Can you work these out from the drawing? Everything is in mm from the part's minimum corner. A direction names the side the tool comes from. Give positions to 0.01 mm unless a question says otherwise; leave off trailing zeros. Order: outer loops, then holes, each group sorted by start corner. A loop starts at its lowest first (then second) coordinate and runs counter-clockwise, first axis right, second up. Notation, with made-up numbers: (12, 20.25) - (16, 20.25) arc R26 cw to (16, 40.25) - close; hole circle Ø9 at (21, -2). An arc over 180 degrees is marked (long way). One line per question, with ' | ' between items.
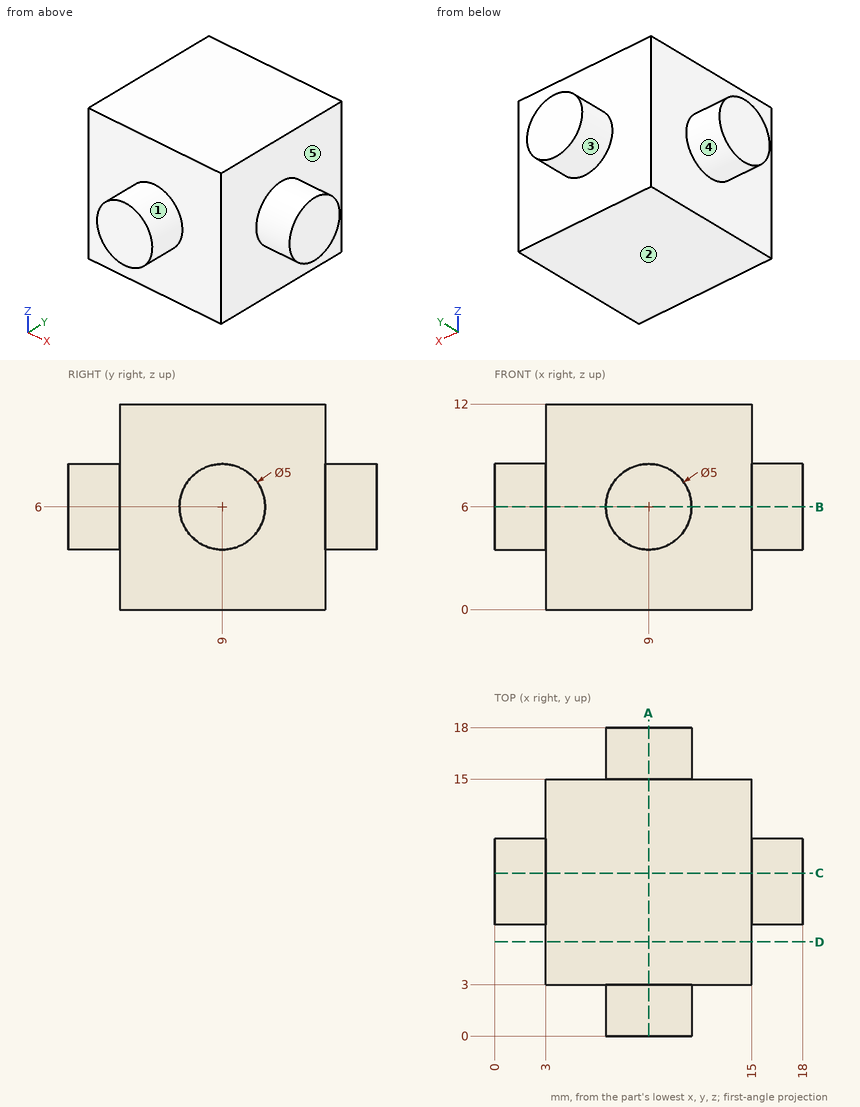
1) On a 3-axis mill with a long thin cutter (end or side, diameter ignored), from which of +Z, -Z, +X, -X, +Y, -Y can I reach the whole of each face in a straight line? I mean the marked faces 1, 2, 3, 4 and 5. Say none if no direction works.
Model answer:
face 1: -Y | face 2: -Z, +X, -X, +Y, -Y | face 3: +Y | face 4: -X | face 5: +X
2) I want a section at C-C (y = 9.5). List the corners of the cut face in (x, z) for me, plus the area to 3 significant figures.
Model answer:
outline: (0, 3.55) - (3, 3.55) - (3, 0) - (15, 0) - (15, 3.55) - (18, 3.55) - (18, 8.45) - (15, 8.45) - (15, 12) - (3, 12) - (3, 8.45) - (0, 8.45) - close | area: 173 mm2
3) I want a section at B-B (z = 6). List the corners of the cut face in (x, y) for me.
Model answer:
outline: (0, 6.5) - (3, 6.5) - (3, 3) - (6.5, 3) - (6.5, 0) - (11.5, 0) - (11.5, 3) - (15, 3) - (15, 6.5) - (18, 6.5) - (18, 11.5) - (15, 11.5) - (15, 15) - (11.5, 15) - (11.5, 18) - (6.5, 18) - (6.5, 15) - (3, 15) - (3, 11.5) - (0, 11.5) - close
4) Please list where these lines run through material, in increasing order: L1, parallel to X at y = 3.5, z = 7.5; L2, parallel to Y at x = 17.25, z = 4.
Model answer:
L1: x = 3 to 15 | L2: y = 7.5 to 10.5
5) I'm going to push flat-ended pins straight in: P1, Ø1.5, axis at y = 2.5, z = 4.5, coming from the -X side; P2, Ø6, axis at x = 11.5, z = 7, coming from the +Y side; P3, Ø1, axis at x = 2, z = 2.5, coming from the -Y side; P4, Ø2, axis at y = 14, z = 3.5, coming from the +X side. Where does each tip first touch, or does it pass through?
Model answer:
P1: stops at x = 3 | P2: stops at y = 18 | P3: passes through | P4: stops at x = 15
6) I want a section at D-D (y = 5.5). List the corners of the cut face in (x, z) for me, plus the area to 3 significant figures.
Model answer:
outline: (3, 0) - (15, 0) - (15, 12) - (3, 12) - close | area: 144 mm2
7) I want a section at A-A (x = 9). List the corners of the cut face in (y, z) for me.
Model answer:
outline: (0, 3.5) - (3, 3.5) - (3, 0) - (15, 0) - (15, 3.5) - (18, 3.5) - (18, 8.5) - (15, 8.5) - (15, 12) - (3, 12) - (3, 8.5) - (0, 8.5) - close
